Design review of the part shown in the three views and the two pictorial views. Dimensions are in mm from the part's minimum x, y and z. A direction names the side the tool comes from. Coordinates: 2 decimals unless noted, no trailing zeros. Loops run counter-clockwise (first coordinate to the right, second up) from the corner with the lowest first, then second, coordinate; pieces in that order, holes last. Notation, with made-up numbers: (79.5, 55.25) -> (125.5, 55.25) arc R8 cw to (125.5, 64.25) -> close; hole circle Ø10 at (83, -33.5). An arc over 180 degrees is marked (long way). Answer in a Markdown table with one row per item.
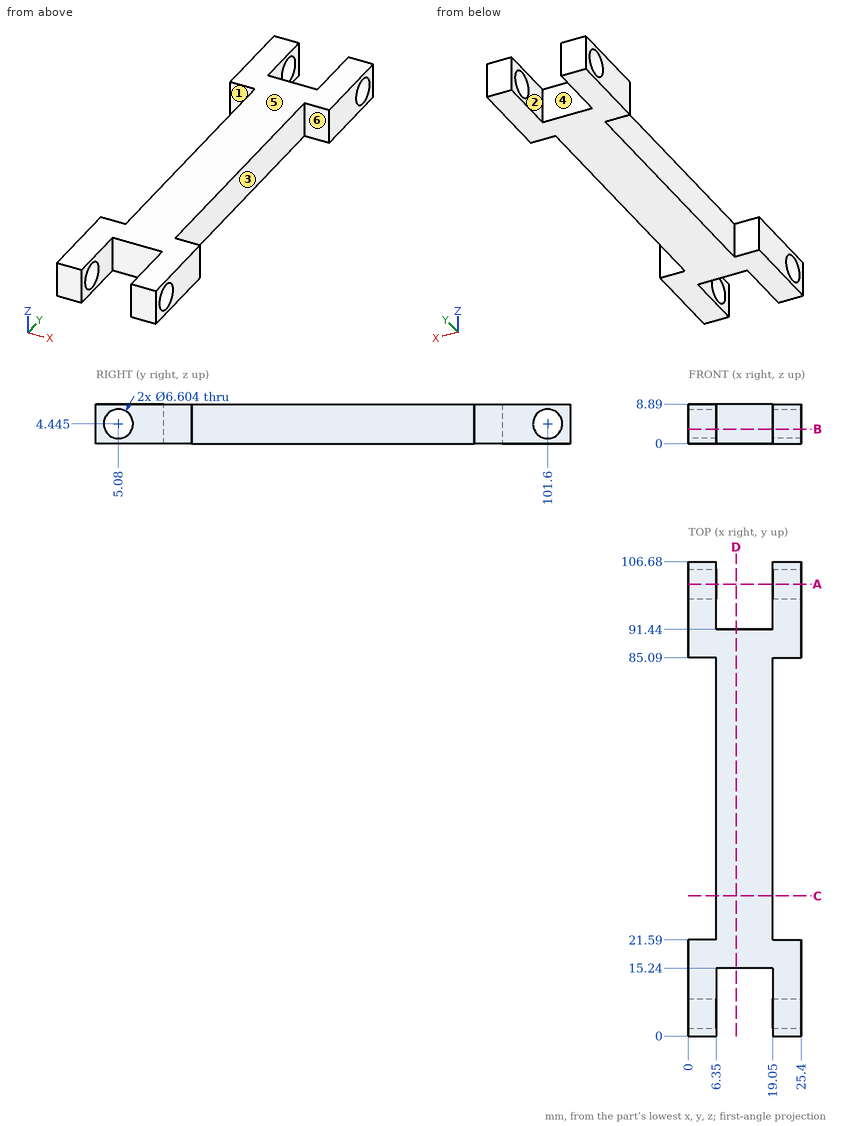
Item 1: For the marked faces 1, 2 and 3, list the 3-axis set-ups (+Z, -Z, +X, -X, +Y, -Y) from which the entire face can be reached by the end or side of a thin tool; tool diameter is ignored.
Worked answers:
| item | result |
|---|---|
| face 1 | +Z, -Z, -X |
| face 2 | +Z, -Z, +Y |
| face 3 | +Z, -Z, +X |
Item 2: Take a section at D-D, the plane x = 10.75. State the section outline as (y, z) points.
Worked answers:
| item | result |
|---|---|
| outline | (15.24, 0) -> (91.44, 0) -> (91.44, 8.89) -> (15.24, 8.89) -> close |
Item 3: Take a section at A-A, the plane y = 101.6. State the section outline as (x, z) points, and give its area (3 significant figures).
Worked answers:
| item | result |
|---|---|
| outline | (0, 0) -> (6.35, 0) -> (6.35, 1.14) -> (0, 1.14) -> close; (0, 7.75) -> (6.35, 7.75) -> (6.35, 8.89) -> (0, 8.89) -> close; (19.05, 0) -> (25.4, 0) -> (25.4, 1.14) -> (19.05, 1.14) -> close; (19.05, 7.75) -> (25.4, 7.75) -> (25.4, 8.89) -> (19.05, 8.89) -> close |
| area | 29.0 mm² |
Item 4: Take a section at C-C, the plane y = 31.5. State the section outline as (x, z) points, and give its area (3 significant figures).
Worked answers:
| item | result |
|---|---|
| outline | (6.35, 0) -> (19.05, 0) -> (19.05, 8.89) -> (6.35, 8.89) -> close |
| area | 113 mm² |
Item 5: For L1, parallel to X at y = 12, z = 2.75; L2, parallel to Y at x = 24, z = 1; L3, parallel to Y at x = 4.5, z = 6, list the stretches that pass through material, from the lowest coordinate up.
Worked answers:
| item | result |
|---|---|
| L1 | 0 to 6.35, 19.05 to 25.4 |
| L2 | 0 to 21.59, 85.09 to 106.68 |
| L3 | 0 to 2.17, 7.99 to 21.59, 85.09 to 98.69, 104.51 to 106.68 |
Item 6: Take a section at B-B, the plane z = 3.25. Count the separate pieces of the cut face and the enclosed holes in it, and give its area (3 significant figures).
Worked answers:
| item | result |
|---|---|
| separate pieces | 5 |
| enclosed holes | 0 |
| area | 1,360 mm² |
Item 7: Insertion check: pin 1 (3 mm diameter, centred on y = 52, z = 5, fed in from -X); pin 2 (1 mm diameter, centred on y = 66.5, z = 7.5, fed in from +X); pin 3 (1 mm diameter, centred on x = 11, z = 2.5, fed in from -Y). Each pin has a flat end and moves straight along its axis. Give the tip position at first contact, or say it passes through.
Worked answers:
| item | result |
|---|---|
| pin 1 | x = 6.35 |
| pin 2 | x = 19.05 |
| pin 3 | y = 15.24 |
Item 8: The part is to be moulded in two halves that separate along Y. For the marked faces 4, 5 and 6, say which applies: +Y half, -Y half, draft (parallel to the pull), parting line (faces both ways), or undercut.
Worked answers:
| item | result |
|---|---|
| face 4 | +Y half |
| face 5 | draft |
| face 6 | undercut |
